from build123d import *

# Parameters (mm, degrees)
ESQUISSE1_W             = 51
ESQUISSE1_H             = 65
BOSS_EXTRU_1_DEPTH      = 5
ESQUISSE2_W             = 5.01
ESQUISSE2_H             = 23.5
ESQUISSE2_H_2           = 24.01
ESQUISSE2_W_2           = 5
ENL_V_MAT_EXTRU_1_DEPTH = 5
ESQUISSE3_W             = 16
ESQUISSE3_H             = 5.07
ESQUISSE3_W_2           = 12
ENL_V_MAT_EXTRU_2_DEPTH = 5


with BuildPart() as part:
    # Esquisse1 → Boss.-Extru.1 (new body)
    with BuildSketch(Plane.XY):
        Rectangle(ESQUISSE1_W, ESQUISSE1_H)
    extrude(amount=BOSS_EXTRU_1_DEPTH)

    # Esquisse2 → Enlèv. mat.-Extru.1 (cut)
    with BuildSketch(Plane.XY.offset(5)):
        with Locations((-22.995, 20.75)):
            Rectangle(ESQUISSE2_W, ESQUISSE2_H)
        with Locations((-22.995, -20.495)):
            Rectangle(ESQUISSE2_W, ESQUISSE2_H_2)
        with Locations((2.005, 20.75)):
            Rectangle(ESQUISSE2_W, ESQUISSE2_H)
        with Locations((2.005, -20.495)):
            Rectangle(ESQUISSE2_W, ESQUISSE2_H_2)
        with Locations((23, 20.75)):
            Rectangle(ESQUISSE2_W_2, ESQUISSE2_H)
        with Locations((23, -20.495)):
            Rectangle(ESQUISSE2_W_2, ESQUISSE2_H_2)
    extrude(amount=-ENL_V_MAT_EXTRU_1_DEPTH, mode=Mode.SUBTRACT)

    # Esquisse3 → Enlèv. mat.-Extru.2 (cut)
    with BuildSketch(Plane.XY.offset(5)):
        with Locations((-17.5, 29.965)):
            Rectangle(ESQUISSE3_W, ESQUISSE3_H)
        with Locations((19.5, 29.965)):
            Rectangle(ESQUISSE3_W_2, ESQUISSE3_H)
        with Locations((19.5, -29.965)):
            Rectangle(ESQUISSE3_W_2, ESQUISSE3_H)
        with Locations((-17.5, -29.965)):
            Rectangle(ESQUISSE3_W, ESQUISSE3_H)
    extrude(amount=-ENL_V_MAT_EXTRU_2_DEPTH, mode=Mode.SUBTRACT)


solid = part.part
The listing builds one solid part. Answer for the finished solid, in the listing's coordinates (mm). A direction names the side the tool comes from. Give positions to 0.01 mm unless a question says otherwise; leave off trailing zeros. Write each loop counter-clockwise with the first axis right and the second up, starting at its lowest first coordinate (ties: lowest second). Pieces come first, ordered by that corner, then holes.
1) Find the intervals of material crossed by L1, parallel to X at y = 20.5, z = 0.8; L2, parallel to X at y = -28.5, z = 3.95; L3, parallel to Y at x = -12, z = 0.3, in increasing order.
2) A tool of negligible diameter and unlimited length cuts with its end or side. For faces 1 (the face through (2, 9, 3)), 2 (the face through (17, -27.43, 3)), 3 (the face through (2, -8.49, 3)), 4 (the face through (-15, 27.43, 3)), 5 (the face through (17, 27.43, 3)), from which of +Z, -Z, +X, -X, +Y, -Y can it reach the whole face along a straight path? Write none if from no direction.
3) Given P1, Ø2.5, axis at x = -23.5, z = 2, coming from the +Y side; P2, Ø2.5, axis at y = 14.5, z = 2.5, coming from the +X side; P3, Ø1.5, axis at x = -12.5, z = 2, coming from the -Y side, each flat-ended and moving along its own axis, determine where each tip first touches the part or whether it passes through.
4) Section A-A (y = 12) is taken. Write down the section's boundary in (x, z).
5) Section C-C (x = 21.5) is taken. Write down the section's boundary in (y, z).
6) Section B-B (z = 2.1) is taken. Write down the section's boundary in (x, y).
Response:
1. L1: x = -20.49 to -0.5, 4.51 to 20.5
1. L2: x = -9.5 to -0.5, 4.51 to 13.5
1. L3: y = -27.43 to 27.43
2. face 1: +Z, -Z, +Y
2. face 2: +Z, -Z, +X, -Y
2. face 3: +Z, -Z, -Y
2. face 4: +Z, -Z, -X, +Y
2. face 5: +Z, -Z, +X, +Y
3. P1: stops at y = 9
3. P2: stops at x = 20.5
3. P3: stops at y = -27.43
4. outline: (-20.49, 0) - (-0.5, 0) - (-0.5, 5) - (-20.49, 5) - close; (4.51, 0) - (20.5, 0) - (20.5, 5) - (4.51, 5) - close
5. outline: (-8.49, 0) - (9, 0) - (9, 5) - (-8.49, 5) - close
6. outline: (-25.5, -8.49) - (-20.49, -8.49) - (-20.49, -27.43) - (-9.5, -27.43) - (-9.5, -32.5) - (-0.5, -32.5) - (-0.5, -8.49) - (4.51, -8.49) - (4.51, -32.5) - (13.5, -32.5) - (13.5, -27.43) - (20.5, -27.43) - (20.5, -8.49) - (25.5, -8.49) - (25.5, 9) - (20.5, 9) - (20.5, 27.43) - (13.5, 27.43) - (13.5, 32.5) - (4.51, 32.5) - (4.51, 9) - (-0.5, 9) - (-0.5, 32.5) - (-9.5, 32.5) - (-9.5, 27.43) - (-20.49, 27.43) - (-20.49, 9) - (-25.5, 9) - close
